Autodesk Inventor part; units mm, degrees
ref_plane "YZ Plane" through (0, 0, 0) normal (1, 0, 0) x (0, 1, 0)
ref_plane "XZ Plane" through (0, 0, 0) normal (0, 1, 0) x (-1, 0, 0)
ref_plane "XY Plane" through (0, 0, 0) normal (0, 0, 1) x (1, 0, 0)
sketch "草图1" plane through (0, 0, 0) normal (0, 1, 0) x (-1, 0, 0)
  circle A0 centre (0, 0) radius 6.5
  dimension "d0" = 13
extrude "拉伸1" add sketch "草图1" along normal blind 44.5
sketch "草图2" plane through (0, 44.5, 0) normal (0, 1, 0) x (1, 0, 0)
  circle A0 centre (0, 0) radius 3
  dimension "d3" = 6
extrude "拉伸2" add sketch "草图2" along normal blind 1
sketch "草图3" plane through (0, 45.5, 0) normal (0, 1, 0) x (1, 0, 0)
  circle A0 centre (0, 0) radius 2.5
  dimension "d6" = 5
extrude "拉伸3" add sketch "草图3" along normal blind 1.5
sketch "草图4" plane through (0, 47, 0) normal (0, 1, 0) x (1, 0, 0)
  circle A0 centre (0, 0) radius 1.5
  dimension "d9" = 3
extrude "拉伸4" add sketch "草图4" along normal blind 7.5
sketch "草图5" plane through (0, 54.5, 0) normal (0, 1, 0) x (1, 0, 0)
  circle A0 centre (0, 0) radius 1.5
  line L0 (0, 0) -> (1, 0)
  line L1 (0, 0) -> (-1, 0)
  line L2 (-1, 0) -> (-1, 1.118)
  circle A1 centre (0, 0) radius 1.5
  line L3 (-1, 0) -> (-1, -1.118)
  line L4 (1, 0) -> (1, -1.118)
  line L5 (1, 0) -> (1, 1.118)
  line L6 (-1, -1.118) -> (-1, 1.118)
  line L7 (1, 1.118) -> (1, -1.118)
  arc A2 (1, -1.118) -> (1, 1.118) centre (0, 0) ccw
  arc A3 (-1, 1.118) -> (-1, -1.118) centre (0, 0) ccw
  dimension "d12" = 1
  dimension "d13" = 1
  dimension "d14" = 1.5
  dimension "d15" = 1.5
extrude "拉伸5" cut sketch "草图5" against normal up to surface (7.5 mm away) contours A0 L4 L5 | L2 L3 A0
sketch "草图6" plane through (0, 44.5, 0) normal (0, 1, 0) x (1, 0, 0)
  circle A0 centre (0, 0) radius 3
  circle A1 centre (0, 0) radius 6.5
  line L0 (0, 0) -> (-4.75, 0)
  line L1 (0, 0) -> (4.75, 0)
  circle A2 centre (-4.75, 0) radius 1
  circle A3 centre (4.75, 0) radius 1
  dimension "d18" = 4.75
  dimension "d19" = 4.75
  dimension "d20" = 2
  dimension "d21" = 2
extrude "拉伸6" cut sketch "草图6" against normal blind 5 contours A2 | A3
properties part number "maxon_motor"
The listing builds one solid part. Answer for the finished solid, in the listing's coordinates (mm). A direction names the side the tool comes from. Round coordinates to 2 decimals unless told otherwise and drop trailing zeros. Loops run counter-clockwise (first coordinate to the right, second up) from the corner with the lowest first, then second, coordinate; pieces in that order, holes last. Notation, with made-up numbers: M -32.5,1 L 2.5,1 A20 ccw 2.5,22 Z; hole C 25.25,-14 d9. An arc over 180 degrees is marked long. Write each question's results on one line, items separated by ' | '. Start each with the question number.
1) Each of these flat-tipped pins is pushed along its axis until it touches: pin 1 (4 mm diameter, centred on x = 2, z = -1, fed in from +Y); pin 2 (2.5 mm diameter, centred on y = 51, z = -0.5, fed in from -X); pin 3 (0.6 mm diameter, centred on x = -4.5, z = 0, fed in from +Y); pin 4 (4 mm diameter, centred on x = 4, y = 32.5, fed in from -Z). Where does it stop, or does it pass through?
2) Find section A-A on z = 0. Write down the section's boundary in (x, y).
3) Find section C-C on y = 19.5. Write down the section's boundary in (x, z), plus the area to 3 significant figures.
4) Which of the six approach directions +Z, -Z, +X, -X, +Y, -Y give full straight-line access (tool end or side, diameter ignored) to faces 5 (the flat face through (-5, 39.5, 0)), 6 (the cylindrical face through (0, 50.7, 1.5)), 7 (the flat face through (1, 51, 0)), 8 (the flat face through (0, 0, 0))?
5) Straight lines are drawn through the part: probe 1 along Y at (x, z) = (4.25, -3); probe 2 along X at (y, z) = (44, 0.5); probe 3 along X at (y, z) = (24, -6). For each, find the intervals that lie inside material, in ascending order.
6) Determine the mould class of faces 1 (the flat face through (-2, 45.5, -2)), 2 (the cylindrical face through (0, 50.7, -1.5)), 3 (the flat face through (-1, 51, 0)), 4 (the cylindrical face through (-5.54, 42.04, 0.61)) for opening direction X: pulls with the +X half, pulls with the -X half, needs draft (parallel to the pull), parting line crosses it, or undercut.
7) Find section B-B on x = 0. Write down the section's boundary in (y, z), plus the area to 4 significant figures.
8) Find section D-D on x = 4.75. Write down the section's boundary in (y, z).
Final values:
1) pin 1: y = 54.5 | pin 2: x = -1 | pin 3: y = 39.5 | pin 4: z = -6.18
2) outline: M -6.5,0 L 6.5,0 L 6.5,44.5 L 5.75,44.5 L 5.75,39.5 L 3.75,39.5 L 3.75,44.5 L 3,44.5 L 3,45.5 L 2.5,45.5 L 2.5,47 L 1,47 L 1,54.5 L -1,54.5 L -1,47 L -2.5,47 L -2.5,45.5 L -3,45.5 L -3,44.5 L -3.75,44.5 L -3.75,39.5 L -5.75,39.5 L -5.75,44.5 L -6.5,44.5 Z
3) outline: C 0,0 d13 | area: 133 mm²
4) face 5: +Y | face 6: +Z, +Y | face 7: +Z, -Z, +X, +Y | face 8: +Z, -Z, +X, -X, -Y
5) probe 1: 0 to 44.5 | probe 2: -6.48 to -5.62, -3.88 to 3.88, 5.62 to 6.48 | probe 3: -2.5 to 2.5
6) face 1: needs draft | face 2: parting line crosses it | face 3: pulls with the -X half | face 4: undercut
7) outline: M 0,-6.5 L 44.5,-6.5 L 44.5,-3 L 45.5,-3 L 45.5,-2.5 L 47,-2.5 L 47,-1.5 L 54.5,-1.5 L 54.5,1.5 L 47,1.5 L 47,2.5 L 45.5,2.5 L 45.5,3 L 44.5,3 L 44.5,6.5 L 0,6.5 Z | area: 614.5 mm²
8) outline: M 0,-4.44 L 44.5,-4.44 L 44.5,-1 L 39.5,-1 L 39.5,1 L 44.5,1 L 44.5,4.44 L 0,4.44 Z
